The model under review builds one solid part; all positions refer to its coordinate system, in mm. Face numbers are marked on the shaded views. A direction names the side the tool comes from. Give positions to 0.01 mm unless a question says otherwise; leave off trailing zeros. Loops run counter-clockwise (first coordinate to the right, second up) from the corner with the lowest first, then second, coordinate; pieces in that order, holes last. Notation, with made-up numbers: (-14, -25) - (14, -25) arc R20 ccw to (14, -20) - close; hole circle Ø4 at (63.25, 80). An arc over 180 degrees is marked (long way). Return JSON: item names as keys, results as strings. Group by question number.
```python
from build123d import *

# Parameters (mm, degrees)
F0_W     = 23
F0_H     = 26
F1_DEPTH = 65.4574409127
F2_R     = 16.367035619
F3_SIZE  = 5.08
F4_T     = -2.5


with BuildPart() as f1:
    # F0 (on Front) → F1 (new body)
    with BuildSketch(Plane.XZ):
        Polygon((-18, 24), (-30, 24), (-30, -30), (40, -30), (40, 24), (5, 24), align=None)
        with Locations((-6.5, 37)):
            Rectangle(F0_W, F0_H)
    extrude(amount=F1_DEPTH)

    # F2
    f2_edges = [f1.edges().sort_by_distance(p)[0] for p in [
        (40, -32.72872, 24),
        (-6.5, -65.457441, 50),
    ]]
    fillet(f2_edges, radius=F2_R)

    # F3
    f3_edges = [f1.edges().sort_by_distance(p)[0] for p in [
        (-30, -65.457441, -3),
    ]]
    chamfer(f3_edges, length=F3_SIZE)

    # F4
    f4_openings = [f1.faces().sort_by_distance(p)[0] for p in [
        (5.094058, -32.641076, -30),
        (-6.5, -24.545203, 50),
        (-6.5, -60.663647, 45.206206),
        (6.241123, -65.457441, -1.444797),
    ]]
    offset(amount=F4_T, openings=f4_openings, kind=Kind.INTERSECTION)


solid = f1.part
```
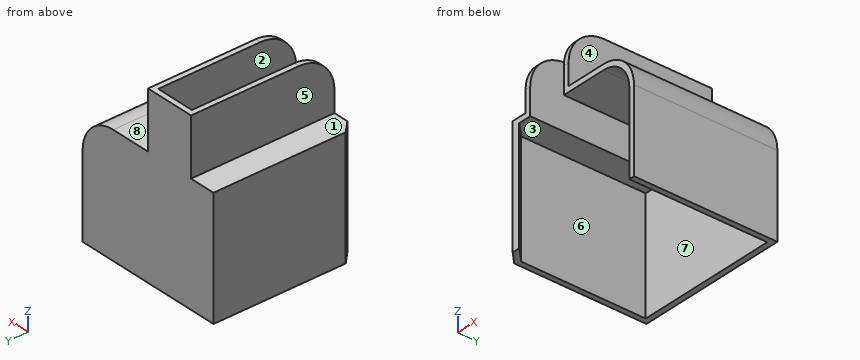
1) We need section A-A, the plane y = -36. Write out the cut boundary in (x, z).
2) We need section D-D, the plane z = 31. Write out the cut boundary in (x, y), plus the area to 3 significant figures.
3) Draft analysis for pull direction X (two halves, no side actions). For the marked faces 5, 6, 7 and 8, state which applies: +X half, -X half, draft (parallel to the pull), parting line (faces both ways), or undercut.
4) For pin 1 Ø8 at (y, z) = (-30, 32.5) entering from -X; pin 2 Ø8.5 at (y, z) = (-26, 38.5) entering from +X; pin 3 Ø5 at (x, y) = (32, -25) entering from -Z; pin 4 Ø8 at (x, y) = (-3, -51.5) entering from -Z, all flat-tipped, find the tip position at first contact; note any pin that passes through.
5) To check wall thickness, follow line 1 (X direction, y = -22.5, z = -8); line 2 (X direction, y = -31, z = 25); line 3 (Z direction, x = 19, y = -61). State the ranges of each line that lie inside material, in increasing order.
6) We need section B-B, the plane z = -18. Write out the cut boundary in (x, y).
7) Tool access review of the marked faces 1, 2, 3 and 4: name each direction out of +Z, -Z, +X, -X, +Y, -Y from which nothing blocks a thin tool from reaching the whole face with its end or side.
8) We need section C-C, the plane x = -23. Write out the cut boundary in (y, z), plus the area to 3 significant figures.
Findings:
{
 "1": {"outline": "(-30, -30) - (-27.5, -30) - (-27.5, 21.5) - (-15.5, 21.5) - (-15.5, 50) - (-18, 50) - (-18, 24) - (-30, 24) - close; (2.5, 21.5) - (23.63, 21.5) arc R13.87 cw to (37.5, 7.63) - (37.5, -30) - (40, -30) - (40, 7.63) arc R16.37 ccw to (23.63, 24) - (5, 24) - (5, 50) - (2.5, 50) - close"},
 "2": {"outline": "(-18, -65.46) - (-15.5, -65.46) - (-15.5, -2.5) - (2.5, -2.5) - (2.5, -65.46) - (5, -65.46) - (5, 0) - (-18, 0) - close", "area": "372 mm^2"},
 "3": {"face 5": "-X half", "face 6": "undercut", "face 7": "undercut", "face 8": "draft"},
 "4": {"pin 1": "stops at x = -18", "pin 2": "stops at x = 5", "pin 3": "stops at z = 16.25", "pin 4": "passes through"},
 "5": {"line 1": "x = -30 to -27.5, 37.5 to 40", "line 2": "x = -18 to -15.5, 2.5 to 5", "line 3": "z = 21.5 to 24"},
 "6": {"outline": "(-30, -60.38) - (-24.92, -65.46) - (-21.38, -65.46) - (-27.5, -59.34) - (-27.5, -2.5) - (37.5, -2.5) - (37.5, -65.46) - (40, -65.46) - (40, 0) - (-30, 0) - close"},
 "7": {"face 1": "+Z, -X, +Y, -Y", "face 2": "+Z, -Z, -Y", "face 3": "-Z", "face 4": "+Z, +X, +Y, -Y"},
 "8": {"outline": "(-65.46, -30) - (-63.84, -30) - (-63.84, 21.5) - (-2.5, 21.5) - (-2.5, -30) - (0, -30) - (0, 24) - (-65.46, 24) - close", "area": "376 mm^2"}
}
